Solid Edge part; units mm, degrees
sketch "Sketch1" plane through (0, 0, 0) normal (0, -1, 0) x (1, 0, 0)
  line L0 (0, 116.4301) -> (0, -14.6322)
  arc A0 (0, 116.43) -> (0, -14.6322) centre (0, 50.8989) cw
revolve "RevolvedProtrusion1" add sketch "Sketch1" angle 360 about axis through (0, 0, 116.4301) along (0, 0, -1)
sketch "Sketch2" plane through (0, 0, 0) normal (0, -1, 0) x (1, 0, 0)
  line L0 (63.9382, 39.399) -> (39.4576, 0)
  line L1 (31.8267, 103.1475) -> (63.9382, 39.399)
  line L2 (-39.5527, 103.1475) -> (31.8267, 103.1475)
  line L3 (-64.0333, 63.7485) -> (-39.5527, 103.1475)
  line L4 (-31.9218, 0) -> (-64.0333, 63.7485)
extrude "Cutout1" cut sketch "Sketch2" along normal mid plane 248 material side at (51.7404, 0, 19.6731)
pattern_circular "Pattern1" count 5 over 360 about axis through (0, 0, 103.1475) along (0, 0, 1) of "Cutout1"
sketch "Sketch3" plane through (0, 0, 0) normal (0, 0, 1) x (1, 0, 0)
  line L0 (-31.9218, -23.1926) -> (12.1931, -37.5264)
  line L1 (12.1931, -37.5264) -> (39.4576, 0)
  line L2 (39.4576, 0) -> (12.1931, 37.5264)
  line L3 (12.1931, 37.5264) -> (-31.9218, 23.1926)
  line L4 (-31.9218, 23.1926) -> (-31.9218, -23.1926)
extrude "ExtrudedCutout_7" cut sketch "Sketch3" against normal blind 58
Check sheet for the modelled part. Datum: model origin and axes. Units: mm. Round coordinates to 2 decimals unless told otherwise and drop trailing zeros. Order: outer loops, then holes, each group sorted by start corner. A loop starts at its lowest first (then second) coordinate and runs counter-clockwise, first axis right, second up. Notation, with made-up numbers: (71, -30.5) - (124, -30.5) arc R18 ccw to (124, -14.5) - close; hole circle Ø8 at (22.5, 3.25). An arc over 180 degrees is marked (long way). Answer as CSV lines item,"result". Start each with the question number.
1) Section check D-D (x = -15). Record the cut outline in (y, z).
2) Section check C-C (y = 17). Record the cut outline in (x, z), then the cut area to 3 significant figures.
3) Scan lines: probe 1 along Y at (x, z) = (13.5, 87); probe 2 along Y at (x, z) = (-24, 92.5); probe 3 along Z at (x, y) = (7.5, -32). Record each from-to range of solid material in increasing order.
4) Section check A-A (z = 37.5). Record the cut outline in (x, y), then the cut area to 3 significant figures.
5) Section check B-B (x = -41). Record the cut outline in (y, z).
6) Depth check by flat-ended pin: pin 1 (12 mm diameter, centred on y = 42.5, z = 13, fed in from +X); pin 2 (8 mm diameter, centred on y = 23.5, z = 88, fed in from -X); pin 3 (8 mm diameter, centred on x = 41.5, z = 67, fed in from -Y). Enter the tip coordinate at first touch or a pass-through.
Determined:
1,outline,"(-60.83, 60.68) - (-28.69, 0) - (28.69, 0) - (60.83, 60.68) - (46.17, 88.37) - (33.5, 103.15) - (-33.5, 103.15) - (-46.17, 88.37) - close"
2,outline,"(-58.44, 52.64) - (-31.92, 0) - (27.11, 0) - (58.44, 50.32) - (31.83, 103.15) - (-26.99, 103.15) - close"
2,area,"9,070 mm^2"
3,probe 1,"-37.63 to 37.63"
3,probe 2,"-30.24 to 30.24"
3,probe 3,"0 to 101.31"
4,outline,"(-50.81, -36.83) - (-50.73, -36.94) - (19.33, -59.71) - (19.46, -59.67) - (62.76, -0.07) - (62.76, 0.07) - (19.46, 59.67) - (19.33, 59.71) - (-50.73, 36.94) - (-50.81, 36.83) - close"
4,area,"9,380 mm^2"
5,outline,"(-45.4, 47.5) - (-29.83, 18.1) - (-29.75, 18.02) - (29.75, 18.02) - (29.83, 18.1) - (45.4, 47.5) - (0, 100.48) - close"
6,pin 1,"x = 22.41"
6,pin 2,"x = -35.52"
6,pin 3,"y = -41.61"
